For this review, take the finished solid that the model builds, in its own axes (mm). Coordinates: 2 decimals unless noted, no trailing zeros. Write each loop counter-clockwise with the first axis right and the second up, starting at its lowest first coordinate (ties: lowest second). Pieces come first, ordered by that corner, then holes. Notation, with made-up numbers: (-32.75, -10) - (26.25, -10) arc R28 ccw to (26.25, 19) - close; hole circle Ø7 at (-28, 29). An arc over 180 degrees is marked (long way). Write each question's results on one line, items separated by ' | '.
from build123d import *

# Parameters (mm, degrees)
F1_DEPTH = 1.5


with BuildPart() as f1:
    # F0 (on Front) → F1 (new body, symmetric)
    with BuildSketch(Plane.XZ):
        with BuildLine():
            Line((0, 87.008731), (0, 237.008731))
            Line((0, 237.008731), (-30, 194.508731))
            Line((-30, 194.508731), (-30, 94.508731))
            Line((-30, 94.508731), (-26, 94.508731))
            Line((-26, 94.508731), (-26, 92.008731))
            Line((-26, 92.008731), (-30, 92.008731))
            Line((-30, 92.008731), (-30, 87.008731))
            Line((-30, 87.008731), (-40, 87.008731))
            Line((-40, 87.008731), (-40, 85.508731))
            ThreePointArc((-40, 85.508731), (-33.034628, 83.570933), (-30, 77.008731))
            Line((-30, 77.008731), (-30, -72.991269))
            Line((-30, -72.991269), (-17.5, -82.991269))
            Line((-17.5, -82.991269), (-12.5, -82.991269))
            Line((-12.5, -82.991269), (0, -72.991269))
            Line((0, -72.991269), (0, 77.008731))
            ThreePointArc((0, 77.008731), (3.036062, 83.565217), (9.999984, 85.491087))
            Line((9.999984, 85.491087), (9.999984, 86.991087))
            Line((9.999984, 86.991087), (0, 87.008731))
        make_face()
        with BuildLine():
            ThreePointArc((-12.5, -79.491269), (-12.792893, -80.198376), (-13.5, -80.491269))
            Line((-13.5, -80.491269), (-16.5, -80.491269))
            ThreePointArc((-16.5, -80.491269), (-17.207107, -80.198376), (-17.5, -79.491269))
            Line((-17.5, -79.491269), (-17.5, -71.491269))
            ThreePointArc((-17.5, -71.491269), (-17.207107, -70.784163), (-16.5, -70.491269))
            Line((-16.5, -70.491269), (-13.5, -70.491269))
            ThreePointArc((-13.5, -70.491269), (-12.792893, -70.784163), (-12.5, -71.491269))
            Line((-12.5, -71.491269), (-12.5, -79.491269))
        make_face(mode=Mode.SUBTRACT)
    extrude(amount=F1_DEPTH, both=True)


solid = f1.part
Q1. For pin 1 (0.9 mm diameter, centred on y = -0.5, z = 172, fed in from +X); pin 2 (0.8 mm diameter, centred on y = -0.5, z = 93, fed in from -X); pin 3 (1.5 mm diameter, centred on y = 0.5, z = 90.5, fed in from -X), all flat-tipped, find the tip position at first contact; note any pin that passes through.
Results found:
pin 1: x = 0 | pin 2: x = -26 | pin 3: x = -30
Q2. Take a section at C-C on x = 5. State the section outline as (y, z) points.
Results found:
outline: (-1.5, 84.82) - (1.5, 84.82) - (1.5, 87) - (-1.5, 87) - close
Q3. Take a section at B-B on z = 72.5. State the section outline as (x, y) points.
Results found:
outline: (-30, -1.5) - (0, -1.5) - (0, 1.5) - (-30, 1.5) - close
Q4. Take a section at A-A on y = -0.8. State the section outline as (x, z) points (1 decimal).
Results found:
outline: (-40, 85.5) arc R8.6 cw to (-30, 77) - (-30, -73) - (-17.5, -83) - (-12.5, -83) - (0, -73) - (0, 77) arc R8.6 cw to (10, 85.5) - (10, 87) - (0, 87) - (0, 237) - (-30, 194.5) - (-30, 94.5) - (-26, 94.5) - (-26, 92) - (-30, 92) - (-30, 87) - (-40, 87) - close; hole (-17.5, -79.5) arc R1 ccw to (-16.5, -80.5) - (-13.5, -80.5) arc R1 ccw to (-12.5, -79.5) - (-12.5, -71.5) arc R1 ccw to (-13.5, -70.5) - (-16.5, -70.5) arc R1 ccw to (-17.5, -71.5) - close
Q5. Wall thickness on line 1 along X through (y, z) = (-1.25, -70); line 2 along Z through (x, y) = (-15.5, -1.25); line 3 along Z through (x, y) = (-16, -0.65): over which ranges is each line inside the solid? List them lowest first. Write a range as from..to.
Results found:
line 1: -30..0 | line 2: -82.99..-80.49, -70.49..215.05 | line 3: -82.99..-80.49, -70.49..214.34
